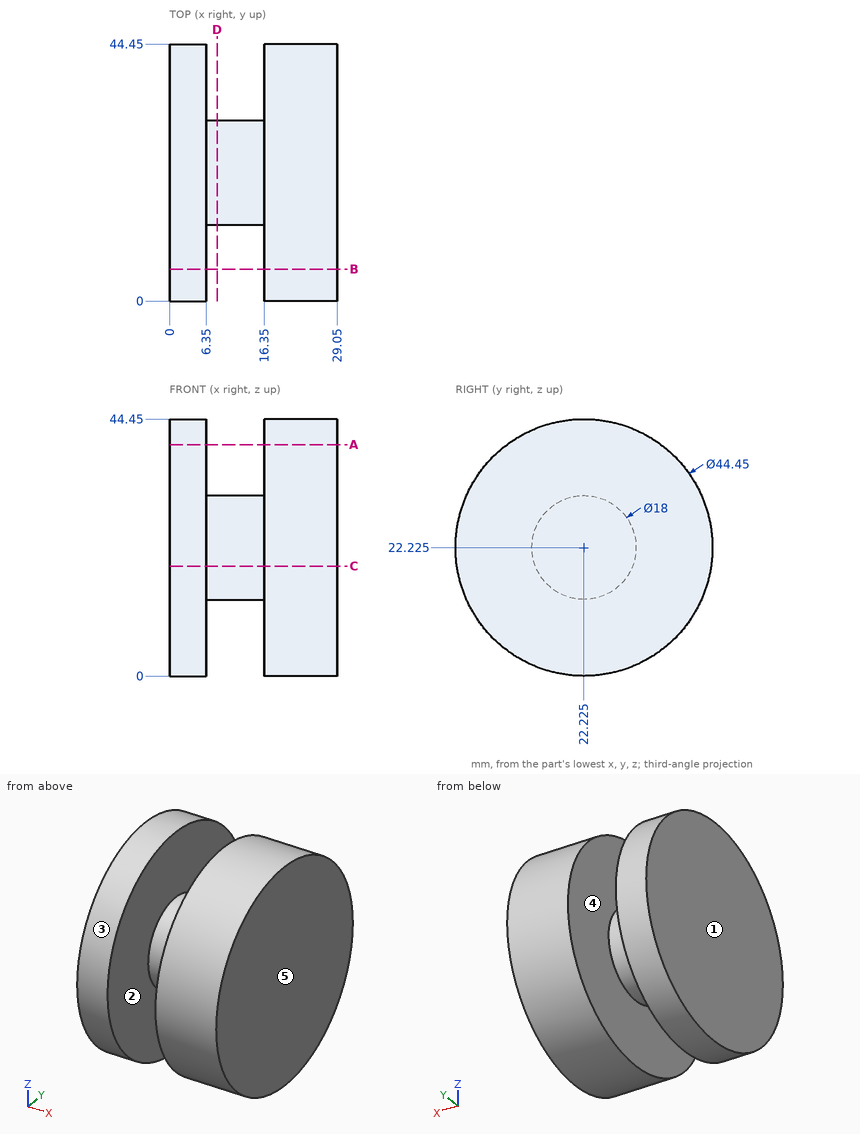
Drawing for the job (mm, zero at the part's lowest x, y, z). A direction names the side the tool comes from. Coordinates: 2 decimals unless noted, no trailing zeros. Order: outer loops, then holes, each group sorted by start corner. A loop starts at its lowest first (then second) coordinate and runs counter-clockwise, first axis right, second up. Notation, with made-up numbers: (-34.75, -16.5) - (16.25, -16.5) arc R9 ccw to (16.25, -5.5) - close; hole circle Ø8 at (14.5, -25.5). An arc over 180 degrees is marked (long way). Use a Markdown table: item, result. Add a question column.
(1) Drill centre lines: line 1 along X through (y, z) = (28, 35); line 2 along Y through (x, z) = (27, 40.5); line 3 along Z through (x, y) = (17.5, 35.5). Where is each one in solid material? Low to high. Write a range as [from, to].
(2) Saw through at D-D (x = 8.25). Give the cut face in (y, z) (3 decimals), then the cut area to 3 significant figures.
(3) Pull direction X, two halves, no side cores. Call the marked faces 3, 4 and 5: +X half, -X half, draft (parallel to the pull), parting line (faces both ways), or undercut.
(4) Flat gauge pins, fed straight in: pin 1 (8 mm diameter, centred on x = 11.5, y = 31, fed in from -Z); pin 2 (1.5 mm diameter, centred on x = 15.5, y = 23, fed in from +Z); pin 3 (3 mm diameter, centred on x = 12, y = 33, fed in from -Z) (1 decimal); pin 4 (6 mm diameter, centred on x = 14.5, z = 28, fed in from -Y). Where does each tip first touch, or does it go through?
(5) Saw through at A-A (z = 40). Give the cut face in (x, y).
(6) Saw through at B-B (y = 5.5). Give the cut face in (x, z).
(7) Saw through at C-C (z = 19). Give the cut face in (x, y), then the cut area to 3 significant figures.
(8) Which spindle directions (+Z, -Z, +X, -X, +Y, -Y) get a long thin tool onto all of the face, cutting with end or side? Do the marked faces 1 and 2. Say none if no direction does.
Solved:
| question | item | result |
|---|---|---|
| 1 | line 1 | x = [0, 6.35], [16.35, 29.05] |
| 1 | line 2 | y = [9.58, 34.87] |
| 1 | line 3 | z = [4.4, 40.05] |
| 2 | outline | circle Ø18 at (22.225, 22.225) |
| 2 | area | 254 mm² |
| 3 | face 3 | draft |
| 3 | face 4 | undercut |
| 3 | face 5 | +X half |
| 4 | pin 1 | stops at z = 14.6 |
| 4 | pin 2 | stops at z = 31.22 |
| 4 | pin 3 | passes through |
| 4 | pin 4 | stops at y = 0.26 |
| 5 | outline | (0, 8.88) - (6.35, 8.88) - (6.35, 35.57) - (0, 35.57) - close; (16.35, 8.88) - (29.05, 8.88) - (29.05, 35.57) - (16.35, 35.57) - close |
| 6 | outline | (0, 7.59) - (6.35, 7.59) - (6.35, 36.86) - (0, 36.86) - close; (16.35, 7.59) - (29.05, 7.59) - (29.05, 36.86) - (16.35, 36.86) - close |
| 7 | outline | (0, 0.24) - (6.35, 0.24) - (6.35, 13.82) - (16.35, 13.82) - (16.35, 0.24) - (29.05, 0.24) - (29.05, 44.21) - (16.35, 44.21) - (16.35, 30.63) - (6.35, 30.63) - (6.35, 44.21) - (0, 44.21) - close |
| 7 | area | 1,010 mm² |
| 8 | face 1 | +Z, -Z, -X, +Y, -Y |
| 8 | face 2 | none |
